```python
from build123d import *

# Parameters (mm, degrees)
F0_R     = 6
F1_DEPTH = 86
F2_W     = 160
F2_H     = 144
F3_DEPTH = 150.001
F4_R     = 6
F5_DEPTH = 150.001


with BuildPart() as f1:
    # F0 (on Front) → F1 (new body, symmetric)
    with BuildSketch(Plane.XZ):
        Polygon((0, 150), (0, 0), (150, 0), (150, 65), (65, 150), align=None)
        with Locations((32.5, 56)):
            Circle(F0_R, mode=Mode.SUBTRACT)
        with Locations((32.5, 126)):
            Circle(F0_R, mode=Mode.SUBTRACT)
    extrude(amount=F1_DEPTH, both=True)

    # F2 (on face) → F3 (cut, through all)
    with BuildSketch(Plane(origin=(0, 0, 0), x_dir=(0, -1, 0), z_dir=(-1, 0, 0))):
        with Locations((0, 78)):
            Rectangle(F2_W, F2_H)
    extrude(amount=-F3_DEPTH, mode=Mode.SUBTRACT)

    # F4 (on face) → F5 (cut, through all)
    with BuildSketch(Plane(origin=(0, 0, 0), x_dir=(1, 0, 0), z_dir=(0, 0, -1))):
        with Locations((110, 40)):
            Circle(F4_R)
        with Locations((110, -40)):
            Circle(F4_R)
        with Locations((30, 40)):
            Circle(F4_R)
        with Locations((30, -40)):
            Circle(F4_R)
    extrude(amount=-F5_DEPTH, mode=Mode.SUBTRACT)


solid = f1.part
```
For this review, take the finished solid that the model builds, in its own axes (mm). A direction names the side the tool comes from. Round coordinates to 2 decimals unless told otherwise and drop trailing zeros. Write each loop counter-clockwise with the first axis right and the second up, starting at its lowest first coordinate (ties: lowest second). Pieces come first, ordered by that corner, then holes. Notation, with made-up numbers: M -29.5,-26.5 L -6.5,-26.5 A27 ccw -6.5,-5.5 Z; hole C -6.75,76 d2. An arc over 180 degrees is marked long. One line per item, written item: value. Start each with the question number.
(1) We need section A-A (z = 75). Give the boundary of the cut face in (x, y).
(2) Insertion check: pin 1 (14 mm diameter, centred on x = 110, y = 40, fed in from +Z); pin 2 (15.5 mm diameter, centred on x = 32.5, z = 126, fed in from +Y). Each pin has a flat end and moves straight along its axis. Give the tip position at first contact, or say it passes through.
(3) We need section B-B (y = -40). Give the boundary of the cut face in (x, z).
(4) Machinability: for faces 1 (the flat face through (74, 1, 6)), 2 (the flat face through (150, 0, 3)), which of the approach directions +Z, -Z, +X, -X, +Y, -Y give a long, thin tool a straight path to every point of the face, cutting with its end or side? Answer none if there is none.
(5) The part is to be moulded in two halves that separate along Z. For faces 3 (the cylindrical face through (27.74, 83.04, 52.35)), 4 (the flat face through (57, -80, 61)), 5 (the flat face through (33, 83, 150)), 6 (the flat face through (74, -1, 0)), say which applies: released by +Z, released by -Z, zero draft, split by the parting line, or undercut.
(6) We need section D-D (z = 126). Give the boundary of the cut face in (x, y).
(7) Wall thickness on line 1 (X direction, y = 40, z = 3.5); line 2 (Z direction, x = 32, y = 84); line 3 (Y direction, x = 30, z = 2.1): over which ranges is each line inside the solid? List them lowest first.
(8) We need section C-C (x = 87.5). Give the boundary of the cut face in (y, z), and give its area (3 significant figures).
Result:
1. outline: M 0,-86 L 140,-86 L 140,-80 L 0,-80 Z; M 0,80 L 140,80 L 140,86 L 0,86 Z
2. pin 1: z = 6
2. pin 2: y = 86
3. outline: M 0,0 L 24,0 L 24,6 L 0,6 Z; M 36,0 L 104,0 L 104,6 L 36,6 Z; M 116,0 L 150,0 L 150,6 L 116,6 Z
4. face 1: +Z, +X, -X
4. face 2: +Z, -Z, +X, +Y, -Y
5. face 3: undercut
5. face 4: zero draft
5. face 5: released by +Z
5. face 6: released by -Z
6. outline: M 0,-86 L 26.5,-86 L 26.5,-80 L 0,-80 Z; M 0,80 L 26.5,80 L 26.5,86 L 0,86 Z; M 38.5,-86 L 89,-86 L 89,-80 L 38.5,-80 Z; M 38.5,80 L 89,80 L 89,86 L 38.5,86 Z
7. line 1: 0 to 24, 36 to 104, 116 to 150
7. line 2: 0 to 50.02, 61.98 to 120.02, 131.98 to 150
7. line 3: -86 to -46, -34 to 34, 46 to 86
8. outline: M -86,0 L 86,0 L 86,127.5 L 80,127.5 L 80,6 L -80,6 L -80,127.5 L -86,127.5 Z
8. area: 2,490 mm²
